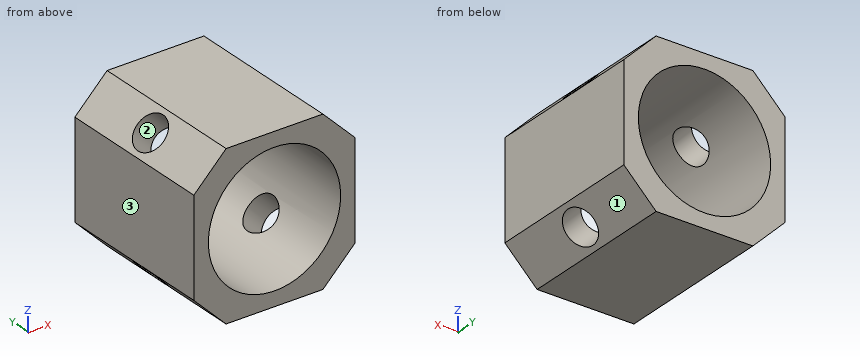
```python
from build123d import *

# Parameters (mm, degrees)
F0_W     = 25
F0_H     = 25
F0_R     = 10.25
F1_DEPTH = 25
F2_SIZE  = 5
F3_R     = 2.75
F4_DEPTH = 31.820805
F5_R     = 2.75
F6_DEPTH = 31.820805


with BuildPart() as f1:
    # F0 (on Front) → F1 (new body)
    with BuildSketch(Plane.XZ):
        Rectangle(F0_W, F0_H)
        Circle(F0_R, mode=Mode.SUBTRACT)
    extrude(amount=F1_DEPTH)

    # F2
    f2_edges = [f1.edges().sort_by_distance(p)[0] for p in [
        (-12.5, -12.5, -12.5),
        (12.5, -12.5, -12.5),
        (12.5, -12.5, 12.5),
        (-12.5, -12.5, 12.5),
    ]]
    chamfer(f2_edges, length=F2_SIZE)

    # F3 (on face) → F4 (cut, through all)
    with BuildSketch(Plane(origin=(10, 0, 10), x_dir=(0, 1, 0), z_dir=(0.707107, 0, 0.707107))):
        with Locations((-12.5, 0)):
            Circle(F3_R)
    extrude(amount=-F4_DEPTH, mode=Mode.SUBTRACT)

    # F5 (on face) → F6 (cut, through all)
    with BuildSketch(Plane(origin=(10, 0, -10), x_dir=(0, 1, 0), z_dir=(0.707107, 0, -0.707107))):
        with Locations((-12.5, 0)):
            Circle(F5_R)
    extrude(amount=-F6_DEPTH, mode=Mode.SUBTRACT)


solid = f1.part
```
Work out the finished part from the listing and answer in its coordinate system (mm). Face numbers are marked on the shaded views. Give positions to 0.01 mm unless a question says otherwise; leave off trailing zeros. Loops run counter-clockwise (first coordinate to the right, second up) from the corner with the lowest first, then second, coordinate; pieces in that order, holes last. Notation, with made-up numbers: (27.25, 37) -> (72.25, 37) arc R34 cw to (72.25, 70) -> close; hole circle Ø6 at (22, 35.25). An arc over 180 degrees is marked (long way). Put each result on its own line as item: value. Start each with the question number.
Item 1: The mould has two halves that part along Z. Classify the marked faces 1, 2 and 3: released by +Z, released by -Z, zero draft, split by the parting line, or undercut.
Item 2: The part is cut by section A-A (z = 0). Give the vertices of the cut face in (x, y), then the cut area to 4 significant figures.
Item 3: The part is cut by section D-D (x = 8.25). State how many separate pieces and enclosed holes the cut face has, then the cut area to 3 significant figures.
Item 4: The part is cut by section C-C (y = -2). Give the vertices of the cut face in (x, z).
Item 5: The part is cut by section B-B (x = 0). Give the vertices of the cut face in (y, z), then the cut area to 4 significant figures.
Item 6: Find the intervals of material crossed by L1, parallel to Z at x = 0, y = -5.5; L2, parallel to Y at x = 7.75, z = 7.75, in increasing order. Write a range as [from, to].
Answers below:
1. face 1: released by -Z
1. face 2: undercut
1. face 3: zero draft
2. outline: (-12.5, -25) -> (-10.25, -25) -> (-10.25, 0) -> (-12.5, 0) -> close; (10.25, -25) -> (12.5, -25) -> (12.5, 0) -> (10.25, 0) -> close
2. area: 112.5 mm2
3. separate pieces: 4
3. enclosed holes: 0
3. area: 228 mm2
4. outline: (-12.5, -7.5) -> (-7.5, -12.5) -> (7.5, -12.5) -> (12.5, -7.5) -> (12.5, 7.5) -> (7.5, 12.5) -> (-7.5, 12.5) -> (-12.5, 7.5) -> close; hole circle Ø20.5 at (0, 0)
5. outline: (-25, -12.5) -> (0, -12.5) -> (0, -10.25) -> (-25, -10.25) -> close; (-25, 10.25) -> (0, 10.25) -> (0, 12.5) -> (-25, 12.5) -> close
5. area: 112.5 mm2
6. L1: [-12.5, -10.25], [10.25, 12.5]
6. L2: [-25, -15.25], [-9.75, 0]
